from build123d import *

# Parameters (mm, degrees)
SKETCH1_W                = 45
SKETCH1_H                = 122
BOSS_EXTRUDE1_DEPTH      = 2.5
SKETCH3_W                = 35
SKETCH3_H                = 2
BOSS_EXTRUDE2_DEPTH      = 15
SKETCH4_W                = 12
SKETCH4_H                = 7
BOSS_EXTRUDE3_DEPTH      = 2.5
SKETCH6_W                = 19
SKETCH6_H                = 100
CUT_EXTRUDE2_DEPTH       = 12.5
FILLET1_SIZE             = 4
SKETCH8_W                = 20
SKETCH8_H                = 15
CUT_EXTRUDE3_DEPTH       = 58.5
FILLET2_SIZE             = 5
SKETCH9_R                = 1.6
CUT_EXTRUDE4_DEPTH       = 58.5
BOSS_EXTRUDE4_DEPTH      = 2.5
BOSS_EXTRUDE4_DEPTH_BACK = 5
SKETCH10_W               = 8
SKETCH10_H               = 5.282493572
SKETCH10_R               = 1.55
BOSS_EXTRUDE5_DEPTH      = 8
BOSS_EXTRUDE6_DEPTH      = 2.5
FILLET3_SIZE             = 2.5
SKETCH13_W               = 15
SKETCH13_H               = 30
CUT_EXTRUDE5_DEPTH       = 6.5
FILLET4_SIZE             = 4
FILLET5_SIZE             = 1
FILLET7_SIZE             = 1


with BuildPart() as part:
    # Sketch1 → Boss-Extrude1 (new body)
    with BuildSketch(Plane(origin=(0, 0, 0), x_dir=(1, 0, 0), z_dir=(0, 1, 0))):
        with Locations((22.5, 61)):
            Rectangle(SKETCH1_W, SKETCH1_H)
    extrude(amount=BOSS_EXTRUDE1_DEPTH)

    # Sketch3 → Boss-Extrude2 (add)
    with BuildSketch(Plane(origin=(0, 2.5, 0), x_dir=(1, 0, 0), z_dir=(0, 1, 0))):
        Polygon((5, 122), (3, 122), (3, 0), (5, 0), (5, 2), align=None)
        with Locations((22.5, 1)):
            Rectangle(SKETCH3_W, SKETCH3_H)
        Polygon((40, 122), (40, 2), (40, 0), (42, 0), (42, 122), align=None)
    extrude(amount=BOSS_EXTRUDE2_DEPTH)

    # Sketch4 → Boss-Extrude3 (add)
    with BuildSketch(Plane(origin=(0, 0, 0), x_dir=(1, 0, 0), z_dir=(0, 1, 0))):
        with Locations((0, 46)):
            Rectangle(SKETCH4_W, SKETCH4_H)
        with Locations((45, 46)):
            Rectangle(SKETCH4_W, SKETCH4_H)
    extrude(amount=BOSS_EXTRUDE3_DEPTH)

    # Sketch6 → Cut-Extrude2 (cut)
    with BuildSketch(Plane(origin=(0, 2.5, 0), x_dir=(1, 0, 0), z_dir=(0, 1, 0))):
        with Locations((22.5, 62)):
            Rectangle(SKETCH6_W, SKETCH6_H)
    extrude(amount=-CUT_EXTRUDE2_DEPTH, mode=Mode.SUBTRACT)

    # Fillet1
    fillet1_edges = [part.edges().sort_by_distance(p)[0] for p in [
        (32, 1.25, -112),
        (32, 1.25, -12),
        (13, 1.25, -12),
        (13, 1.25, -112),
    ]]
    chamfer(fillet1_edges, length=FILLET1_SIZE)

    # Sketch8 → Cut-Extrude3 (cut)
    with BuildSketch(Plane(origin=(51, 0, 0), x_dir=(0, 0, -1), z_dir=(1, 0, 0))):
        with Locations((46, 10)):
            Rectangle(SKETCH8_W, SKETCH8_H)
    extrude(amount=-CUT_EXTRUDE3_DEPTH, mode=Mode.SUBTRACT)

    # Fillet2
    fillet2_edges = [part.edges().sort_by_distance(p)[0] for p in [
        (4, 17.5, -56),
        (41, 17.5, -56),
        (4, 2.5, -36),
        (41, 2.5, -36),
        (4, 17.5, -36),
        (41, 17.5, -36),
        (4, 2.5, -56),
        (41, 2.5, -56),
        (4, 17.5, -122),
        (41, 17.5, -122),
    ]]
    chamfer(fillet2_edges, length=FILLET2_SIZE)

    # Sketch9 → Cut-Extrude4 (cut)
    with BuildSketch(Plane.XZ):
        with Locations(Location((48.5, -46, 0), (0, 0, 270))):
            Circle(SKETCH9_R)
        with Locations(Location((-3.5, -46, 0), (0, 0, 270))):
            Circle(SKETCH9_R)
    extrude(amount=-CUT_EXTRUDE4_DEPTH, mode=Mode.SUBTRACT)



with BuildPart() as body_2:
    # Sketch10 → Boss-Extrude4 (new, two sides: drawn at the far end of the back side and taken through both)
    with BuildSketch(Plane(origin=(0, 0, 0), x_dir=(1, 0, 0), z_dir=(0, 1, 0)).offset(-BOSS_EXTRUDE4_DEPTH_BACK)):
        with Locations((22.5, 124.641246786)):
            Rectangle(SKETCH10_W, SKETCH10_H)
        with Locations(Location((22.5, 124.641246786, 0), (0, 0, 270))):
            Circle(SKETCH10_R, mode=Mode.SUBTRACT)
    extrude(amount=BOSS_EXTRUDE4_DEPTH + BOSS_EXTRUDE4_DEPTH_BACK)


with BuildPart() as part_1:
    add(part.part)

    add(body_2.part)  # Boss-Extrude5 merges body 2
    # Sketch11 → Boss-Extrude5 (add)
    with BuildSketch(Plane.ZY.offset(-18.5)):
        Polygon((-119.5, 0), (-122.028446462, -2.5), (-122, 0), align=None)
    extrude(amount=-BOSS_EXTRUDE5_DEPTH)

    # Sketch12 → Boss-Extrude6 (add)
    with BuildSketch(Plane(origin=(0, 2.5, 0), x_dir=(1, 0, 0), z_dir=(0, 1, 0))):
        Polygon((18.5, 127.282493572), (18.5, 122), (13.22, 122), align=None)
        Polygon((26.5, 122), (31.78, 122), (26.5, 127.282493572), align=None)
    extrude(amount=-BOSS_EXTRUDE6_DEPTH)

    # Fillet3
    # the kernel refuses this chamfer: 2.5 mm, written as the material it adds along each edge
    with BuildSketch(Plane(origin=(26.5, 0, -113.07079253), x_dir=(0.9996219169112968, 0.027495876610586372, 0), z_dir=(0, 0, -1))) as fillet3_piece_1_section:
        Polygon((FILLET3_SIZE * 0.999621916911, FILLET3_SIZE * 0.0274958766106), (-FILLET3_SIZE * 0.0274958766106, FILLET3_SIZE * 0.999621916911), (0, 0), align=None)
    fillet3_piece_1 = extrude(amount=14.211701041, mode=Mode.PRIVATE)
    fillet3_piece_1 = split(fillet3_piece_1, bisect_by=Plane(origin=(26.425464868, -2.516462273, -122.045096052), z_dir=(0, -0.7110955817269744, 0.7030953517470985)), keep=Keep.TOP, mode=Mode.PRIVATE)
    fillet3_piece_1 = split(fillet3_piece_1, bisect_by=Plane(origin=(26.425464868, -2.531550229, -122), z_dir=(0, 0, -1)), keep=Keep.TOP, mode=Mode.PRIVATE)
    add(fillet3_piece_1)
    with BuildSketch(Plane(origin=(26.5, 0, -113.07079253), x_dir=(0.9996219169112968, 0.027495876610586372, 0), z_dir=(0, 0, -1))) as fillet3_piece_2_section:
        Polygon((FILLET3_SIZE * 0.999621916911, FILLET3_SIZE * 0.0274958766106), (-FILLET3_SIZE * 0.0274958766106, FILLET3_SIZE * 0.999621916911), (0, 0), align=None)
    fillet3_piece_2 = extrude(amount=14.211701041, mode=Mode.PRIVATE)
    fillet3_piece_2 = split(fillet3_piece_2, bisect_by=Plane(origin=(27.453210407, -1.061082343, -120.573155958), z_dir=(0, 0.7110955817269744, -0.7030953517470985)), keep=Keep.TOP, mode=Mode.PRIVATE)
    fillet3_piece_2 = split(fillet3_piece_2, bisect_by=Plane(origin=(27.453210407, -0.58369775, -122), z_dir=(0, 0, 1)), keep=Keep.TOP, mode=Mode.PRIVATE)
    add(fillet3_piece_2)
    with BuildSketch(Plane(origin=(26.5, 0, -113.07079253), x_dir=(0.9996219169112968, 0.027495876610586372, 0), z_dir=(0, 0, -1))) as fillet3_piece_3_section:
        Polygon((FILLET3_SIZE * 0.999621916911, FILLET3_SIZE * 0.0274958766106), (-FILLET3_SIZE * 0.0274958766106, FILLET3_SIZE * 0.999621916911), (0, 0), align=None)
    fillet3_piece_3 = extrude(amount=14.211701041, mode=Mode.PRIVATE)
    fillet3_piece_3 = split(fillet3_piece_3, bisect_by=Plane(origin=(27.235712014, -2.816950005, -122.349002909), z_dir=(0, 0.7110955817269744, -0.7030953517470985)), keep=Keep.TOP, mode=Mode.PRIVATE)
    fillet3_piece_3 = split(fillet3_piece_3, bisect_by=Plane(origin=(28.372764332, -0.871738969, -125.408844794), z_dir=(-0.7072736937748051, 0, 0.7069398291892623)), keep=Keep.TOP, mode=Mode.PRIVATE)
    fillet3_piece_3 = split(fillet3_piece_3, bisect_by=Plane(origin=(27.235712014, -0.871738969, -122), z_dir=(0, 0, -1)), keep=Keep.TOP, mode=Mode.PRIVATE)
    add(fillet3_piece_3)
    with BuildSketch(Plane(origin=(18.5, 0, -127.282493572), x_dir=(0.027495876610586317, -0.9996219169112968, 0), z_dir=(0, 0, 1))) as fillet3_piece_4_section:
        Polygon((FILLET3_SIZE * 0.999621916911, -FILLET3_SIZE * 0.0274958766106), (-FILLET3_SIZE * 0.0274958766106, -FILLET3_SIZE * 0.999621916911), (0, 0), align=None)
    fillet3_piece_4 = extrude(amount=14.211701041, mode=Mode.PRIVATE)
    fillet3_piece_4 = split(fillet3_piece_4, bisect_by=Plane(origin=(17.764287986, -2.816950005, -122.349002909), z_dir=(0, 0.7110955817269744, -0.7030953517470985)), keep=Keep.TOP, mode=Mode.PRIVATE)
    fillet3_piece_4 = split(fillet3_piece_4, bisect_by=Plane(origin=(17.764287986, -0.871738969, -122), z_dir=(0, 0, -1)), keep=Keep.TOP, mode=Mode.PRIVATE)
    fillet3_piece_4 = split(fillet3_piece_4, bisect_by=Plane(origin=(16.627235668, -0.871738969, -125.408844794), z_dir=(0.7072736937748045, 0, 0.7069398291892628)), keep=Keep.TOP, mode=Mode.PRIVATE)
    add(fillet3_piece_4)
    with BuildSketch(Plane(origin=(18.5, 0, -127.282493572), x_dir=(0.027495876610586317, -0.9996219169112968, 0), z_dir=(0, 0, 1))) as fillet3_piece_5_section:
        Polygon((FILLET3_SIZE * 0.999621916911, -FILLET3_SIZE * 0.0274958766106), (-FILLET3_SIZE * 0.0274958766106, -FILLET3_SIZE * 0.999621916911), (0, 0), align=None)
    fillet3_piece_5 = extrude(amount=14.211701041, mode=Mode.PRIVATE)
    fillet3_piece_5 = split(fillet3_piece_5, bisect_by=Plane(origin=(17.546789593, -1.061082343, -120.573155958), z_dir=(0, 0.7110955817269744, -0.7030953517470985)), keep=Keep.TOP, mode=Mode.PRIVATE)
    fillet3_piece_5 = split(fillet3_piece_5, bisect_by=Plane(origin=(17.546789593, -0.58369775, -122), z_dir=(0, 0, 1)), keep=Keep.TOP, mode=Mode.PRIVATE)
    add(fillet3_piece_5)
    with BuildSketch(Plane(origin=(18.5, 0, -127.282493572), x_dir=(0.027495876610586317, -0.9996219169112968, 0), z_dir=(0, 0, 1))) as fillet3_piece_6_section:
        Polygon((FILLET3_SIZE * 0.999621916911, -FILLET3_SIZE * 0.0274958766106), (-FILLET3_SIZE * 0.0274958766106, -FILLET3_SIZE * 0.999621916911), (0, 0), align=None)
    fillet3_piece_6 = extrude(amount=14.211701041, mode=Mode.PRIVATE)
    fillet3_piece_6 = split(fillet3_piece_6, bisect_by=Plane(origin=(18.574535132, -2.516462273, -122.045096052), z_dir=(0, -0.7110955817269744, 0.7030953517470985)), keep=Keep.TOP, mode=Mode.PRIVATE)
    fillet3_piece_6 = split(fillet3_piece_6, bisect_by=Plane(origin=(18.574535132, -2.531550229, -122), z_dir=(0, 0, -1)), keep=Keep.TOP, mode=Mode.PRIVATE)
    add(fillet3_piece_6)

    # Sketch13 → Cut-Extrude5 (cut)
    with BuildSketch(Plane.XY):
        with Locations((22.5, 17.5)):
            Rectangle(SKETCH13_W, SKETCH13_H)
    extrude(amount=-CUT_EXTRUDE5_DEPTH, mode=Mode.SUBTRACT)

    # Fillet4
    fillet4_edges = [part_1.edges().sort_by_distance(p)[0] for p in [
        (30, 17.5, -1),
        (15, 17.5, -1),
        (30, 2.5, -1),
        (15, 2.5, -1),
    ]]
    chamfer(fillet4_edges, length=FILLET4_SIZE)

    # Fillet5
    fillet5_edges = [part_1.edges().sort_by_distance(p)[0] for p in [
        (42, 2.5, -20.5),
        (3, 2.5, -20.5),
        (3, 2.5, -86.5),
        (42, 2.5, -86.5),
    ]]
    chamfer(fillet5_edges, length=FILLET5_SIZE)

    # Fillet7
    fillet7_edges = [part_1.edges().sort_by_distance(p)[0] for p in [
        (-6, 1.25, -42.5),
        (-6, 1.25, -49.5),
        (51, 1.25, -49.5),
        (51, 1.25, -42.5),
    ]]
    chamfer(fillet7_edges, length=FILLET7_SIZE)


solid = part_1.part
Work out the finished part from the listing and answer in its coordinate system (mm). A direction names the side the tool comes from. Coordinates: 2 decimals unless noted, no trailing zeros. Loops run counter-clockwise (first coordinate to the right, second up) from the corner with the lowest first, then second, coordinate; pieces in that order, holes last. Notation, with made-up numbers: M 23.5,-8 L 66.5,-8 A26 ccw 66.5,7 Z; hole C -16.75,63.5 d8. An arc over 180 degrees is marked long. Answer in a Markdown table with one row per item. Add a question column.
1. Consider L1, parallel to X at y = 1.15, z = -46; L2, parallel to X at y = 2, z = -93.5; L3, parallel to X at y = 9.5, z = -97. Determine where each line is inside the solid, lowest interval first.
2. Flat-ended cylindrical pins translate along their axes: P1, Ø0.8, axis at y = -3.5, z = -125.5, coming from the +X side; P2, Ø7, axis at x = 31, y = 9.5, coming from the -Z side; P3, Ø4, axis at y = 15, z = -61.5, coming from the +X side; P4, Ø4, axis at x = 6.5, y = -2.5, coming from the -Z side. Find the tip coordinate at first contact, or state that the pin passes through.
3. Find section B-B, the plane z = -46. Write down the section's boundary in (x, y).
4. Find section D-D, the plane y = 10.25. Write down the section's boundary in (x, z).
5. A tool of negligible diameter and unlimited length cuts with its end or side. For faces 4 (the flat face through (3, 10, -87)), 5 (the flat face through (41.2, 5, -38.5)), 6 (the flat face through (42, 10, -20)), 7 (the flat face through (13, 1, -61)), from which of +Z, -Z, +X, -X, +Y, -Y can it reach the whole face along a straight path? Write none if from no direction.
6. Find section C-C, the plane x = -3.5. Write down the section's boundary in (y, z), then the cut area to 3 significant figures.
7. Find section A-A, the plane x = 22.5. Write down the section's boundary in (y, z), then the cut area to 3 significant figures.
8. The mould has two halves that part along Z. Classify faces 1 (the flat face through (0, 1, -21)), 2 (the flat face through (23, -4, -122)), 3 (the flat face through (30, 1, -110)): pulls with the +Z half, pulls with the -Z half, needs draft (parallel to the pull), parting line crosses it, or undercut.
Reported:
| question | item | result |
|---|---|---|
| 1 | L1 | x = -6 to -5.1, -1.9 to 13, 32 to 46.9, 50.1 to 51 |
| 1 | L2 | x = 0 to 13, 32 to 45 |
| 1 | L3 | x = 3 to 5, 40 to 42 |
| 2 | P1 | stops at x = 26.5 |
| 2 | P2 | stops at z = -2 |
| 2 | P3 | stops at x = 42 |
| 2 | P4 | passes through |
| 3 | outline | M -6,0 L -5.1,0 L -5.1,2.5 L -6,2.5 Z; M -1.9,0 L 13,0 L 13,2.5 L -1.9,2.5 Z; M 32,0 L 46.9,0 L 46.9,2.5 L 32,2.5 Z; M 50.1,0 L 51,0 L 51,2.5 L 50.1,2.5 Z |
| 4 | outline | M 3,-122 L 5,-122 L 5,-56 L 3,-56 Z; M 3,-36 L 5,-36 L 5,-2 L 15,-2 L 15,0 L 3,0 Z; M 30,-2 L 40,-2 L 40,-36 L 42,-36 L 42,0 L 30,0 Z; M 40,-122 L 42,-122 L 42,-56 L 40,-56 Z |
| 5 | face 4 | +Z, -Z, -X, +Y |
| 5 | face 5 | +X, -X, +Y |
| 5 | face 6 | +Z, -Z, +X, +Y |
| 5 | face 7 | +Y, -Y |
| 6 | outline | M 0,-49.5 L 2.5,-49.5 L 2.5,-47.6 L 0,-47.6 Z; M 0,-44.4 L 2.5,-44.4 L 2.5,-42.5 L 0,-42.5 Z |
| 6 | area | 9.50 mm^2 |
| 7 | outline | M -5,-127.28 L 2.5,-127.28 L 2.5,-126.19 L -5,-126.19 Z; M -5,-123.09 L 2.5,-123.09 L 2.5,-112 L 0,-112 L 0,-119.5 L -2.47,-122 L -5,-122 Z; M 0,-12 L 2.5,-12 L 2.5,0 L 0,0 Z |
| 7 | area | 74.5 mm^2 |
| 8 | face 1 | needs draft |
| 8 | face 2 | pulls with the +Z half |
| 8 | face 3 | undercut |
